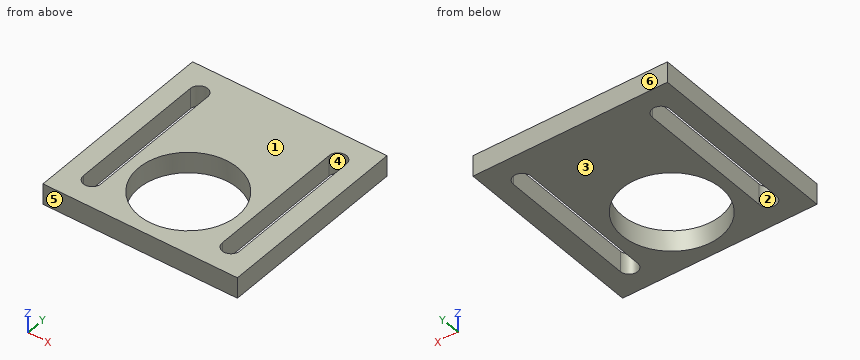
from build123d import *

# Parameters (mm, degrees)
SKETCH1_W           = 56
SKETCH1_H           = 56
BOSS_EXTRUDE1_DEPTH = 6
SKETCH2_R           = 14.275
CUT_EXTRUDE1_DEPTH  = 6


with BuildPart() as part:
    # Sketch1 → Boss-Extrude1 (new body)
    with BuildSketch(Plane.XY):
        with Locations((28, 28)):
            Rectangle(SKETCH1_W, SKETCH1_H)
    extrude(amount=BOSS_EXTRUDE1_DEPTH)

    # Sketch2 → Cut-Extrude1 (cut)
    with BuildSketch(Plane.XY.offset(6)):
        with Locations((28, 18)):
            Circle(SKETCH2_R)
        with BuildLine():
            Line((10.5, 48), (10.5, 8))
            ThreePointArc((10.5, 8), (8, 5.5), (5.5, 8))
            Line((5.5, 8), (5.5, 48))
            ThreePointArc((5.5, 48), (8, 50.5), (10.5, 48))
        make_face()
        with BuildLine():
            Line((50.5, 48), (50.5, 8))
            ThreePointArc((50.5, 8), (48, 5.5), (45.5, 8))
            Line((45.5, 8), (45.5, 48))
            ThreePointArc((45.5, 48), (48, 50.5), (50.5, 48))
        make_face()
    extrude(amount=-CUT_EXTRUDE1_DEPTH, mode=Mode.SUBTRACT)


solid = part.part
Geometry check sheet. Reference: the model listing, model coordinates, mm. Face numbers are marked on the shaded views. A direction names the side the tool comes from. Round coordinates to 2 decimals unless told otherwise and drop trailing zeros. Loops run counter-clockwise (first coordinate to the right, second up) from the corner with the lowest first, then second, coordinate; pieces in that order, holes last.
Item 1: Gauge pin test, flat end, axial feed: pin 1 (3 mm diameter, centred on y = 23, z = 3.5, fed in from -X). Record the tip position at first contact, or that the pin passes through.
Item 2: Cross-section at B-B on x = 8. Record the boundary of the cut face in (y, z).
Item 3: Cross-section at A-A on y = 36. Record the boundary of the cut face in (x, z).
Item 4: Thickness scan on line 1 (X direction, y = 36, z = 2.3); line 2 (Y direction, x = 48, z = 0.5); line 3 (Y direction, x = 28, z = 1.6) (3 decimals). Record the ranges inside material, lowest first.
Item 5: Cross-section at D-D on y = 18. Record the boundary of the cut face in (x, z) (3 decimals).
Item 6: Cross-section at C-C on z = 1.85. Record the boundary of the cut face in (x, y) (3 decimals).
Item 7: Mould release check, pull along Y, two halves, no side actions. Record for the marked faces 3, 4, 5 and 6: pulls with the +Y half, pulls with the -Y half, needs draft (parallel to the pull), parting line crosses it, or undercut.
Item 8: Access from +Z, -Z, +X, -X, +Y, -Y to the whole of each face (thin tool, end or side, straight path). Record for the marked faces 1 and 2.
Answer sheet:
1. pin 1: stops at x = 0
2. outline: (0, 0) - (5.5, 0) - (5.5, 6) - (0, 6) - close; (50.5, 0) - (56, 0) - (56, 6) - (50.5, 6) - close
3. outline: (0, 0) - (5.5, 0) - (5.5, 6) - (0, 6) - close; (10.5, 0) - (45.5, 0) - (45.5, 6) - (10.5, 6) - close; (50.5, 0) - (56, 0) - (56, 6) - (50.5, 6) - close
4. line 1: x = 0 to 5.5, 10.5 to 45.5, 50.5 to 56
4. line 2: y = 0 to 5.5, 50.5 to 56
4. line 3: y = 0 to 3.725, 32.275 to 56
5. outline: (0, 0) - (5.5, 0) - (5.5, 6) - (0, 6) - close; (10.5, 0) - (13.725, 0) - (13.725, 6) - (10.5, 6) - close; (42.275, 0) - (45.5, 0) - (45.5, 6) - (42.275, 6) - close; (50.5, 0) - (56, 0) - (56, 6) - (50.5, 6) - close
6. outline: (0, 0) - (56, 0) - (56, 56) - (0, 56) - close; hole (5.5, 8) arc R2.5 ccw to (10.5, 8) - (10.5, 48) arc R2.5 ccw to (5.5, 48) - close; hole circle Ø28.55 at (28, 18); hole (45.5, 8) arc R2.5 ccw to (50.5, 8) - (50.5, 48) arc R2.5 ccw to (45.5, 48) - close
7. face 3: needs draft
7. face 4: undercut
7. face 5: pulls with the -Y half
7. face 6: pulls with the +Y half
8. face 1: +Z, +X, -X, +Y, -Y
8. face 2: +Z, -Z
